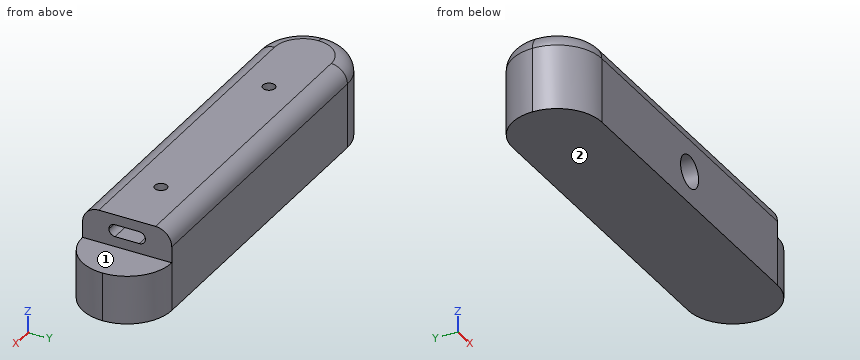
from build123d import *

# Parameters (mm, degrees)
SKETCH_1_W          = 100
SKETCH_1_H          = 22
EXTRUDE_3_DEPTH     = 20
CUT_EXTRUDE_2_DEPTH = 20
CUT_EXTRUDE_3_DEPTH = 8
SKETCH_5_W          = 3
SKETCH_5_H          = 9
CUT_EXTRUDE_5_DEPTH = 7
EXTRUDE_4_DEPTH     = 7
SKETCH_8_R          = 6
CUT_EXTRUDE_7_DEPTH = 10
FILLET_1_R          = 4
SKETCH_9_R          = 1.5
CUT_EXTRUDE_8_DEPTH = 5
SKETCH_10_R         = 6
EXTRUDE_5_DEPTH     = 10
SKETCH_11_R         = 4
CUT_EXTRUDE_9_DEPTH = 10


with BuildPart() as part:
    # Sketch 1 → Extrude 3 (new body)
    with BuildSketch(Plane.XY):
        Rectangle(SKETCH_1_W, SKETCH_1_H)
    extrude(amount=EXTRUDE_3_DEPTH)

    # Sketch 3 → Cut-Extrude 2 (cut)
    with BuildSketch(Plane.XY.offset(20)):
        with BuildLine():
            ThreePointArc((-50, 0), (-46.778174593, 7.778174593), (-39, 11))
            Line((-39, 11), (-50, 11))
            Line((-50, 11), (-50, 0))
        make_face()
        with BuildLine():
            ThreePointArc((-39, -11), (-46.778174593, -7.778174593), (-50, 0))
            Line((-50, 0), (-50, -11))
            Line((-50, -11), (-39, -11))
        make_face()
        with BuildLine():
            Line((50, -11), (50, 0))
            ThreePointArc((50, 0), (46.778174593, -7.778174593), (39, -11))
            Line((39, -11), (50, -11))
        make_face()
        with BuildLine():
            Line((50, 11), (39, 11))
            ThreePointArc((39, 11), (46.778174593, 7.778174593), (50, 0))
            Line((50, 0), (50, 11))
        make_face()
    extrude(amount=-CUT_EXTRUDE_2_DEPTH, mode=Mode.SUBTRACT)

    # Sketch 4 → Cut-Extrude 3 (cut)
    with BuildSketch(Plane.XY.offset(20)):
        with BuildLine():
            Line((39, 11), (39, -11))
            ThreePointArc((39, -11), (50, 0), (39, 11))
        make_face()
    extrude(amount=-CUT_EXTRUDE_3_DEPTH, mode=Mode.SUBTRACT)

    # Sketch 5 → Cut-Extrude 5 (cut)
    with BuildSketch(Plane(origin=(39, 0, 0), x_dir=(0, 0, -1), z_dir=(1, 0, 0))):
        with Locations((-16, 0)):
            Rectangle(SKETCH_5_W, SKETCH_5_H)
    extrude(amount=-CUT_EXTRUDE_5_DEPTH, mode=Mode.SUBTRACT)

    # Sketch 7 → Extrude 4 (add)
    with BuildSketch(Plane(origin=(32, 0, 0), x_dir=(0, 0, -1), z_dir=(1, 0, 0))):
        with BuildLine():
            ThreePointArc((-17.5, 3), (-17.060660172, 4.060660172), (-16, 4.5))
            Line((-16, 4.5), (-17.5, 4.5))
            Line((-17.5, 4.5), (-17.5, 3))
        make_face()
        with BuildLine():
            Line((-14.5, 4.5), (-16, 4.5))
            ThreePointArc((-16, 4.5), (-14.939339828, 4.060660172), (-14.5, 3))
            Line((-14.5, 3), (-14.5, 4.5))
        make_face()
        with BuildLine():
            Line((-14.5, -4.5), (-14.5, -3))
            ThreePointArc((-14.5, -3), (-14.939339828, -4.060660172), (-16, -4.5))
            Line((-16, -4.5), (-14.5, -4.5))
        make_face()
        with BuildLine():
            ThreePointArc((-16, -4.5), (-17.060660172, -4.060660172), (-17.5, -3))
            Line((-17.5, -3), (-17.5, -4.5))
            Line((-17.5, -4.5), (-16, -4.5))
        make_face()
    extrude(amount=EXTRUDE_4_DEPTH)

    # Sketch 8 → Cut-Extrude 7 (cut)
    with BuildSketch(Plane.XZ.offset(11)):
        with Locations(Location((0, 10, 0), (0, 0, 270))):
            Circle(SKETCH_8_R)
    extrude(amount=-CUT_EXTRUDE_7_DEPTH, mode=Mode.SUBTRACT)

    # Fillet 1
    fillet_1_edges = [part.edges().sort_by_distance(p)[0] for p in [
        (0, 11, 20),
        (-50, 0, 20),
        (0, -11, 20),
    ]]
    fillet(fillet_1_edges, radius=FILLET_1_R - 0.0001)  # a hair under: the kernel refuses the full size

    # Sketch 9 → Cut-Extrude 8 (cut)
    with BuildSketch(Plane.XY.offset(20)):
        with Locations((-24, 0)):
            Circle(SKETCH_9_R)
        with Locations(Location((24, 0, 0), (0, 0, 180))):
            Circle(SKETCH_9_R)
    extrude(amount=-CUT_EXTRUDE_8_DEPTH, mode=Mode.SUBTRACT)

    # Sketch 10 → Extrude 5 (add)
    with BuildSketch(Plane.XZ.offset(11)):
        with Locations((0, 10)):
            Circle(SKETCH_10_R)
    extrude(amount=-EXTRUDE_5_DEPTH)

    # Sketch 11 → Cut-Extrude 9 (cut)
    with BuildSketch(Plane.XZ.offset(11)):
        with Locations(Location((0, 8, 0), (0, 0, 270))):
            Circle(SKETCH_11_R)
    extrude(amount=-CUT_EXTRUDE_9_DEPTH, mode=Mode.SUBTRACT)


solid = part.part
Design review of the part built by this model. Coordinates are the model's own, in mm. Face numbers are marked on the shaded views. A direction names the side the tool comes from. Round coordinates to 2 decimals unless told otherwise and drop trailing zeros. Write each loop counter-clockwise with the first axis right and the second up, starting at its lowest first coordinate (ties: lowest second). Pieces come first, ordered by that corner, then holes. Notation, with made-up numbers: (6.25, 2.25) - (12.25, 2.25) arc R31 cw to (12.25, 41.25) - close; hole circle Ø5 at (-25.75, -31). An arc over 180 degrees is marked (long way). Return JSON: item names as keys, results as strings. Group by question number.
Item 1: We need section B-B on z = 8. Write out the cut boundary in (x, y), and give its area (3 significant figures).
Item 2: For probe 1 along Y at (x, z) = (-39.5, 8.25); probe 2 along Z at (x, y) = (-37, -7.25); probe 3 along Z at (x, y) = (-3, -8), list the stretches that pass through material, from the lowest coordinate up. Write a range as [from, to].
Item 3: Insertion check: P1, Ø7, axis at x = 0, z = 8, coming from the -Y side; P2, Ø2.5, axis at y = -2.5, z = 16.5, coming from the +X side; P3, Ø0.9, axis at y = 1, z = 16.5, coming from the +X side. Each pin has a flat end and moves straight along its axis. Give the tip position at first contact, or say it passes through.
Item 4: We need section A-A on x = 24. Write out the cut boundary in (y, z), and give its area (3 significant figures).
Item 5: Machinability: for the marked faces 1 and 2, which of the approach directions +Z, -Z, +X, -X, +Y, -Y give a long, thin tool a straight path to every point of the face, cutting with its end or side? Answer none if there is none.
Item 6: We need section D-D on x = -32.5. Write out the cut boundary in (y, z).
Item 7: We need section C-C on x = 0. Write out the cut boundary in (y, z), and give its area (3 significant figures).
Model answer:
{
 "1": {"outline": "(-39, -11) - (-4, -11) - (-4, -1) - (4, -1) - (4, -11) - (39, -11) arc R11 ccw to (39, 11) - (-39, 11) arc R11 ccw to start", "area": "2,020 mm²"},
 "2": {"probe 1": "y = [-10.99, 10.99]", "probe 2": "z = [0, 19.99]", "probe 3": "z = [0, 5.35], [10.65, 19.87]"},
 "3": {"P1": "stops at y = -1", "P2": "stops at x = 39", "P3": "stops at x = 32"},
 "4": {"outline": "(-11, 0) - (11, 0) - (11, 16) arc R4 ccw to (7, 20) - (1.5, 20) - (1.5, 15) - (-1.5, 15) - (-1.5, 20) - (-7, 20) arc R4 ccw to (-11, 16) - close", "area": "418 mm²"},
 "5": {"face 1": "+Z, +X, +Y, -Y", "face 2": "-Z, +X, -X, +Y, -Y"},
 "6": {"outline": "(-11, 0) - (11, 0) - (11, 16) arc R4 ccw to (7, 20) - (-7, 20) arc R4 ccw to (-11, 16) - close"},
 "7": {"outline": "(-11, 0) - (11, 0) - (11, 16) arc R4 ccw to (7, 20) - (-7, 20) arc R4 ccw to (-11, 16) - (-11, 12) - (-1, 12) - (-1, 4) - (-11, 4) - close", "area": "353 mm²"}
}
